Work out the finished part from the listing and answer in its coordinate system (mm). A direction names the side the tool comes from. Round coordinates to 2 decimals unless told otherwise and drop trailing zeros. Loops run counter-clockwise (first coordinate to the right, second up) from the corner with the lowest first, then second, coordinate; pieces in that order, holes last. Notation, with made-up numbers: (-31, -2.75) - (14, -2.75) arc R25 cw to (14, 17.25) - close; hole circle Ø4 at (2, -35.5). An arc over 180 degrees is marked (long way). Return JSON: item names as keys, results as strings.
from build123d import *

# Parameters (mm, degrees)
SKETCH1_W                                           = 70
SKETCH1_H                                           = 55
BOSS_EXTRUDE1_DEPTH                                 = 74
CUT_EXTRUDE1_DEPTH                                  = 116.762688289
CUT_EXTRUDE1_DEPTH_BACK                             = 116.762688289
SKETCH4_R                                           = 1.25
CUT_EXTRUDE4_DEPTH                                  = 7
SKETCH5_W                                           = 14.985710671
SKETCH5_H                                           = 55
CUT_EXTRUDE5_DEPTH                                  = 63
CSK_FOR_M3_COUNTERSUNK_FLAT_HEAD_SCREW1_D           = 3.4
CSK_FOR_M3_COUNTERSUNK_FLAT_HEAD_SCREW1_DEPTH       = 10
CSK_FOR_M3_COUNTERSUNK_FLAT_HEAD_SCREW1_CSINK_D     = 6.3
CSK_FOR_M3_COUNTERSUNK_FLAT_HEAD_SCREW1_CSINK_ANGLE = 90
CSK_FOR_M3_COUNTERSUNK_FLAT_HEAD_SCREW1_TIP         = 1.021463052


with BuildPart() as part:
    # Sketch1 → Boss-Extrude1 (new body)
    with BuildSketch(Plane.XY):
        with Locations((35, 27.5)):
            Rectangle(SKETCH1_W, SKETCH1_H)
    extrude(amount=BOSS_EXTRUDE1_DEPTH)

    # Sketch2 → Cut-Extrude1 (cut, two sides: drawn at the far end of the back side and taken through both)
    with BuildSketch(Plane.XY.offset(74).offset(-CUT_EXTRUDE1_DEPTH_BACK)):
        Polygon((7, 0), (7, 45), (63, 45), (63, 15), (70, 15), (70, 0), (60, 0), align=None)
    extrude(amount=CUT_EXTRUDE1_DEPTH + CUT_EXTRUDE1_DEPTH_BACK, mode=Mode.SUBTRACT)

    # Sketch4 → Cut-Extrude4 (cut)
    with BuildSketch(Plane(origin=(70, 0, 0), x_dir=(0, 0, -1), z_dir=(1, 0, 0))):
        with Locations((-83.331764561, 40)):
            Circle(SKETCH4_R)
        with Locations((-75.331764561, 20)):
            Circle(SKETCH4_R)
        with Locations(Location((-62.331764561, 40, 0), (0, 0, 90))):
            Circle(SKETCH4_R)
        with Locations(Location((-54.331764561, 20, 0), (0, 0, 90))):
            Circle(SKETCH4_R)
        with Locations(Location((-41.331764561, 40, 0), (0, 0, 90))):
            Circle(SKETCH4_R)
        with Locations(Location((-33.331764561, 20, 0), (0, 0, 90))):
            Circle(SKETCH4_R)
        with Locations(Location((-20.331764561, 40, 0), (0, 0, 90))):
            Circle(SKETCH4_R)
        with Locations(Location((-12.331764561, 20, 0), (0, 0, 90))):
            Circle(SKETCH4_R)
    extrude(amount=-CUT_EXTRUDE4_DEPTH, mode=Mode.SUBTRACT)

    # Sketch5 → Cut-Extrude5 (cut)
    with BuildSketch(Plane.ZY):
        with Locations((7.492855336, 27.5)):
            Rectangle(SKETCH5_W, SKETCH5_H)
        with Locations((66.507144665, 27.5)):
            Rectangle(SKETCH5_W, SKETCH5_H)
    extrude(amount=-CUT_EXTRUDE5_DEPTH, mode=Mode.SUBTRACT)

    # CSK for M3 Countersunk Flat Head Screw1
    with Locations(Plane(origin=(7, 0, 0), x_dir=(0, 0, 1), z_dir=(1, 0, 0))):
        with Locations((23.167654473, -38.739261213), (23.167654473, -13.339261213), (51.107654473, -13.339261213), (51.107654473, -38.739261213)):
            CounterSinkHole(CSK_FOR_M3_COUNTERSUNK_FLAT_HEAD_SCREW1_D / 2, CSK_FOR_M3_COUNTERSUNK_FLAT_HEAD_SCREW1_CSINK_D / 2, depth=CSK_FOR_M3_COUNTERSUNK_FLAT_HEAD_SCREW1_DEPTH, counter_sink_angle=CSK_FOR_M3_COUNTERSUNK_FLAT_HEAD_SCREW1_CSINK_ANGLE)
            with Locations((0, 0, -(CSK_FOR_M3_COUNTERSUNK_FLAT_HEAD_SCREW1_DEPTH + CSK_FOR_M3_COUNTERSUNK_FLAT_HEAD_SCREW1_TIP / 2))):  # 118° drill point
                Cone(0, CSK_FOR_M3_COUNTERSUNK_FLAT_HEAD_SCREW1_D / 2, CSK_FOR_M3_COUNTERSUNK_FLAT_HEAD_SCREW1_TIP, mode=Mode.SUBTRACT)


solid = part.part
1) Section B-B (y = 29) is taken. Give the vertices of the cut face in (x, z), and give its area (3 significant figures).
Verdict:
{"outline": "(0, 14.99) - (7, 14.99) - (7, 59.01) - (0, 59.01) - close; (63, 0) - (70, 0) - (70, 74) - (63, 74) - close", "area": "826 mm2"}
2) Section A-A (y = 20) is taken. Give the vertices of the cut face in (x, z).
Verdict:
{"outline": "(0, 14.99) - (7, 14.99) - (7, 59.01) - (0, 59.01) - close; (63, 0) - (70, 0) - (70, 11.08) - (63, 11.08) - close; (63, 13.58) - (70, 13.58) - (70, 32.08) - (63, 32.08) - close; (63, 34.58) - (70, 34.58) - (70, 53.08) - (63, 53.08) - close; (63, 55.58) - (70, 55.58) - (70, 74) - (63, 74) - close"}
3) Find the intervals of material crossed by L1, parallel to Z at x = 66, y = 40; L2, parallel to Z at x = 64.5, y = 20; L3, parallel to X at y = 35, z = 32.5, in increasing order.
Verdict:
{"L1": "z = 0 to 19.08, 21.58 to 40.08, 42.58 to 61.08, 63.58 to 74", "L2": "z = 0 to 11.08, 13.58 to 32.08, 34.58 to 53.08, 55.58 to 74", "L3": "x = 0 to 7, 63 to 70"}
4) Determine the mould class of faces 1 (the cylindrical face through (66.55, 39.73, 61.11)), 2 (the flat face through (66, 35, 0)), 3 (the flat face through (35, 45, 37)) for opening direction Z: pulls with the +Z half, pulls with the -Z half, needs draft (parallel to the pull), parting line crosses it, or undercut.
Verdict:
{"face 1": "undercut", "face 2": "pulls with the -Z half", "face 3": "needs draft"}
5) Flat-ended cylindrical pins translate along their axes: pin 1 (4 mm diameter, centred on y = 40, z = 62.33, fed in from -X); pin 2 (2 mm diameter, centred on x = 66, z = 34, fed in from -Y); pin 3 (16.5 mm diameter, centred on x = 34, y = 33.5, fed in from -Z); pin 4 (10 mm diameter, centred on y = 9, z = 47.5, fed in from +X). Find the tip coordinate at first contact, or state that the pin passes through.
Verdict:
{"pin 1": "stops at x = 63", "pin 2": "stops at y = 15", "pin 3": "passes through", "pin 4": "stops at x = 7"}
6) Section D-D (y = 46.5) is taken. Give the vertices of the cut face in (x, z).
Verdict:
{"outline": "(0, 14.99) - (63, 14.99) - (63, 0) - (70, 0) - (70, 74) - (63, 74) - (63, 59.01) - (0, 59.01) - close"}
7) A tool of negligible diameter and unlimited length cuts with its end or side. For faces 4 (the flat face through (22, 46, 14.986)), 5 (the cylindrical face through (66.55, 39.73, 40.11)), 6 (the flat face through (66, 15, 36)), 7 (the flat face through (7, 22, 37)), 8 (the cylindrical face through (2.736, 39.39, 49.537)), from which of +Z, -Z, +X, -X, +Y, -Y can it reach the whole face along a straight path? Write none if from no direction.
Verdict:
{"face 4": "-Z, -X, +Y, -Y", "face 5": "+X", "face 6": "+Z, -Z, +X, -Y", "face 7": "+Z, -Z, -Y", "face 8": "-X"}
8) Section C-C (z = 39) is taken. Give the vertices of the cut face in (x, y).
Verdict:
{"outline": "(0, 0) - (7, 0) - (7, 45) - (63, 45) - (63, 15) - (70, 15) - (70, 55) - (0, 55) - close"}
